```python
from build123d import *

# Parameters (mm, degrees)
SKETCH1_R                          = 4.7625
SKETCH1_R_2                        = 2.86564839
SKETCH1_R_3                        = 3.16650189
BOSS_EXTRUDE1_DEPTH                = 6.35
TAP_DRILL_FOR_6_32_TAP1_AT_2_COUNT = 2
TAP_DRILL_FOR_6_32_TAP1_AT_2_PITCH = 9.525


with BuildPart() as part:
    # Sketch1 → Boss-Extrude1 (new body)
    with BuildSketch(Plane.XY):
        Polygon((25.4, -11.1125), (25.4, -12.7), (-25.4, -12.7), (-25.4, -11.1125), (-19.05, -11.1125), (-19.05, 11.1125), (-25.4, 11.1125), (-25.4, 12.7), (25.4, 12.7), (25.4, 11.1125), (19.05, 11.1125), (19.05, -11.1125), align=None)
        Circle(SKETCH1_R, mode=Mode.SUBTRACT)
        with Locations((-10.863100334, 0)):
            Circle(SKETCH1_R_2, mode=Mode.SUBTRACT)
        with Locations((10.650098366, 0)):
            Circle(SKETCH1_R_3, mode=Mode.SUBTRACT)
    extrude(amount=BOSS_EXTRUDE1_DEPTH)

    # Sketch4 → Tap Drill for #6-32 Tap1 (revolve, cut)
    with BuildSketch(Plane(origin=(19.05, 4.7625, 3.175), x_dir=(0, 0, -1), z_dir=(0, 1, 0))):
        Polygon((0, 0), (0, 7.16269403), (1.35255, 6.35), (1.35255, 0), align=None)
    tap_drill_for_6_32_tap1 = revolve(axis=Axis((25.4, 4.7625, 3.175), (-1, 0, 0)), mode=Mode.SUBTRACT)

    # Tap Drill for #6-32 Tap1 at 2: Tap Drill for #6-32 Tap1 ×2
    with Locations(*[(0, -i * TAP_DRILL_FOR_6_32_TAP1_AT_2_PITCH, 0) for i in range(1, TAP_DRILL_FOR_6_32_TAP1_AT_2_COUNT)]):
        add(tap_drill_for_6_32_tap1, mode=Mode.SUBTRACT)

    # Mirror1: Tap Drill for #6-32 Tap1 across plane
    add(tap_drill_for_6_32_tap1.mirror(Plane.ZY), mode=Mode.SUBTRACT)

    # Mirror1 copy 1 sketch → Mirror1 copy 1 (revolve, cut)
    with BuildSketch(Plane(origin=(-19.05, -4.7625, 3.175), x_dir=(0, 0, -1), z_dir=(0, 1, 0))):
        Polygon((0, 0), (0, -7.16269403), (1.35255, -6.35), (1.35255, 0), align=None)
    revolve(axis=Axis((-25.4, -4.7625, 3.175), (-1, 0, 0)), mode=Mode.SUBTRACT)


solid = part.part
```
Work out the finished part from the listing and answer in its coordinate system (mm). A direction names the side the tool comes from. Coordinates: 2 decimals unless noted, no trailing zeros. Write each loop counter-clockwise with the first axis right and the second up, starting at its lowest first coordinate (ties: lowest second). Pieces come first, ordered by that corner, then holes. Notation, with made-up numbers: (8, 51) - (64, 51) arc R14 ccw to (64, 56) - close; hole circle Ø3 at (-22, -4). An arc over 180 degrees is marked (long way). Answer as a JSON object with one key per item and string values.
Q1. Find section B-B (y = 0). Write down the section's boundary in (x, z).
Results list:
{"outline": "(-19.05, 0) - (-13.73, 0) - (-13.73, 6.35) - (-19.05, 6.35) - close; (-8, 0) - (-4.76, 0) - (-4.76, 6.35) - (-8, 6.35) - close; (4.76, 0) - (7.48, 0) - (7.48, 6.35) - (4.76, 6.35) - close; (13.82, 0) - (19.05, 0) - (19.05, 6.35) - (13.82, 6.35) - close"}
Q2. Consider L1, parallel to X at y = 0.5, z = 4; L2, parallel to Y at x = 14, z = 4; L3, parallel to Y at x = -17, z = 2. Determine where each line is inside the solid, lowest interval first. Write a range as from..to.
Results list:
{"L1": "x = -19.05..-13.68, -8.04..-4.74, 4.74..7.52, 13.78..19.05", "L2": "y = -12.7..-5.83, -3.69..3.69, 5.83..12.7", "L3": "y = -12.7..-5.43, -4.09..4.09, 5.43..12.7"}
Q3. Find section C-C (z = 5.5). State how many separate pieces and enclosed holes the cut face has, plus the area to 3 significant figures.
Results list:
{"separate pieces": "1", "enclosed holes": "3", "area": "880 mm^2"}
Q4. Find section A-A (x = -22). Write down the section's boundary in (y, z).
Results list:
{"outline": "(-12.7, 0) - (-11.11, 0) - (-11.11, 6.35) - (-12.7, 6.35) - close; (11.11, 0) - (12.7, 0) - (12.7, 6.35) - (11.11, 6.35) - close"}
Q5. For a pull along X with two mould halves and no side action, classify faces 1 (the conical face through (-12.03, -5, 3.21)), 2 (the flat face through (19.05, 0, 3)), 3 (the cylindrical face through (-3.78, -2.9, 3.13)), 4 (the flat face through (-22, -11.112, 3)) as pulls with the +X half, pulls with the -X half, needs draft (parallel to the pull), parting line crosses it, or undercut.
Results list:
{"face 1": "pulls with the -X half", "face 2": "pulls with the +X half", "face 3": "undercut", "face 4": "needs draft"}
Q6. Given pin 1 Ø3 at (y, z) = (-4.76, 3.18) entering from +X; pin 2 Ø1 at (x, y) = (-7, 9.5) entering from -Z; pin 3 Ø1 at (y, z) = (-3.5, 4.5) entering from -X; pin 4 Ø1.6 at (y, z) = (4.76, 3.18) entering from +X, each flat-ended and moving along its own axis, determine where each tip first touches the part or whether it passes through.
Results list:
{"pin 1": "stops at x = 19.05", "pin 2": "stops at z = 0", "pin 3": "stops at x = -19.05", "pin 4": "stops at x = 12.37"}
Q7. Find section D-D (x = 0). Write down the section's boundary in (y, z).
Results list:
{"outline": "(-12.7, 0) - (-4.76, 0) - (-4.76, 6.35) - (-12.7, 6.35) - close; (4.76, 0) - (12.7, 0) - (12.7, 6.35) - (4.76, 6.35) - close"}
Q8. Which of the six approach directions +Z, -Z, +X, -X, +Y, -Y give full straight-line access (tool end or side, diameter ignored) to faces 5 (the cylindrical face through (-15.919, -4.822, 4.526)), 6 (the cylindrical face through (15.919, -4.822, 4.526)), 7 (the flat face through (22, 11.112, 3)), 8 (the flat face through (-19.05, 0, 3))?
Results list:
{"face 5": "-X", "face 6": "+X", "face 7": "+Z, -Z, +X", "face 8": "+Z, -Z, -X"}
